Source: three-view drawing plus pictorial views. Frame: mm from the lowest corner of the part. Give positions to 0.01 mm unless a question says otherwise; leave off trailing zeros. Loops run counter-clockwise (first coordinate to the right, second up) from the corner with the lowest first, then second, coordinate; pieces in that order, holes last. Notation, with made-up numbers: (71, 1.25) - (103, 1.25) arc R17 cw to (103, 26.25) - close; hole circle Ø9 at (66.5, 9). An arc over 180 degrees is marked (long way). Answer as a JSON object with one key per item and string values.
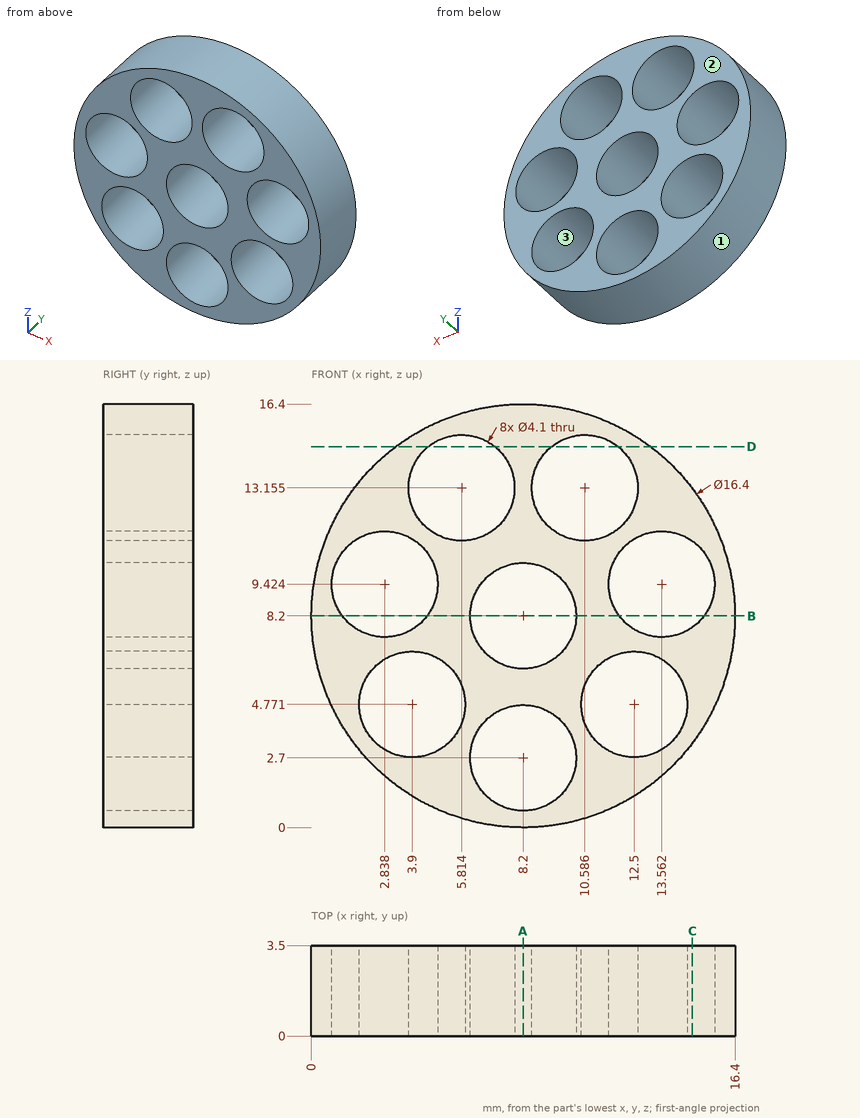
Item 1: Cut plane C-C (x = 14.75). Return loops of the section in (y, z) (1 decimal).
Geometry check:
{"outline": "(0, 3.3) - (3.5, 3.3) - (3.5, 7.8) - (0, 7.8) - close; (0, 11.1) - (3.5, 11.1) - (3.5, 13.1) - (0, 13.1) - close"}
Item 2: Cut plane B-B (z = 8.2). Return loops of the section in (x, y).
Geometry check:
{"outline": "(0, 0) - (1.19, 0) - (1.19, 3.5) - (0, 3.5) - close; (4.48, 0) - (6.15, 0) - (6.15, 3.5) - (4.48, 3.5) - close; (10.25, 0) - (11.92, 0) - (11.92, 3.5) - (10.25, 3.5) - close; (15.21, 0) - (16.4, 0) - (16.4, 3.5) - (15.21, 3.5) - close"}
Item 3: Material intervals for line 1 (Z direction, x = 8.2, y = 2.1); line 2 (X direction, y = 1.1, z = 6.5) (1 decimal); line 3 (Z direction, x = 2.75, y = 1.4) (1 decimal), sorted ascending. Write a range as [from, to].
Geometry check:
{"line 1": "z = [0, 0.65], [4.75, 6.15], [10.25, 16.4]", "line 2": "x = [0.2, 2.8], [5, 7.1], [9.3, 11.4], [13.6, 16.2]", "line 3": "z = [2.1, 3.1], [6.5, 7.4], [11.5, 14.3]"}
Item 4: Mould query, pull axis X, two halves, no side actions, for the marked faces 1, 2 and 3. Classes: released by +X, released by -X, zero draft, split by the parting line, or undercut.
Geometry check:
{"face 1": "split by the parting line", "face 2": "zero draft", "face 3": "undercut"}
Item 5: Cut plane D-D (z = 14.75). Return loops of the section in (x, y) (1 decimal), then the cut area to 3 significant figures.
Geometry check:
{"outline": "(3.3, 0) - (4.5, 0) - (4.5, 3.5) - (3.3, 3.5) - close; (7.1, 0) - (9.3, 0) - (9.3, 3.5) - (7.1, 3.5) - close; (11.9, 0) - (13.1, 0) - (13.1, 3.5) - (11.9, 3.5) - close", "area": "16.5 mm2"}
Item 6: Cut plane A-A (x = 8.2). Return loops of the section in (y, z), then the cut area to 3 significant figures.
Geometry check:
{"outline": "(0, 0) - (3.5, 0) - (3.5, 0.65) - (0, 0.65) - close; (0, 4.75) - (3.5, 4.75) - (3.5, 6.15) - (0, 6.15) - close; (0, 10.25) - (3.5, 10.25) - (3.5, 16.4) - (0, 16.4) - close", "area": "28.7 mm2"}
